```python
from build123d import *

# Parameters (mm, degrees)
SKETCH1_W           = 90
SKETCH1_H           = 30
SKETCH1_R           = 10.585
BOSS_EXTRUDE1_DEPTH = 80
SKETCH2_W           = 90
SKETCH2_H           = 30
BOSS_EXTRUDE2_DEPTH = 5
SKETCH3_W           = 90
SKETCH3_H           = 30
BOSS_EXTRUDE3_DEPTH = 5
SKETCH4_W           = 81.17
SKETCH4_H           = 74
CUT_EXTRUDE1_DEPTH  = 15


with BuildPart() as part:
    # Sketch1 → Boss-Extrude1 (new body)
    with BuildSketch(Plane(origin=(0, 0, 0), x_dir=(1, 0, 0), z_dir=(0, 1, 0))):
        with Locations((30, 0)):
            Rectangle(SKETCH1_W, SKETCH1_H)
        with Locations(Location((0, 0, 0), (0, 0, 270))):
            Circle(SKETCH1_R, mode=Mode.SUBTRACT)
        with Locations(Location((60, 0, 0), (0, 0, 270))):
            Circle(SKETCH1_R, mode=Mode.SUBTRACT)
        with Locations(Location((30, 0, 0), (0, 0, 270))):
            Circle(SKETCH1_R, mode=Mode.SUBTRACT)
    extrude(amount=BOSS_EXTRUDE1_DEPTH)

    # Sketch2 → Boss-Extrude2 (add)
    with BuildSketch(Plane(origin=(0, 80, 0), x_dir=(1, 0, 0), z_dir=(0, 1, 0))):
        with Locations((30, 0)):
            Rectangle(SKETCH2_W, SKETCH2_H)
    extrude(amount=BOSS_EXTRUDE2_DEPTH)

    # Sketch3 → Boss-Extrude3 (add)
    with BuildSketch(Plane.XZ):
        with Locations((30, 0)):
            Rectangle(SKETCH3_W, SKETCH3_H)
    extrude(amount=BOSS_EXTRUDE3_DEPTH)

    # Sketch4 → Cut-Extrude1 (cut)
    with BuildSketch(Plane(origin=(0, 0, -15), x_dir=(-1, 0, 0), z_dir=(0, 0, -1))):
        with Locations((-30, 40)):
            Rectangle(SKETCH4_W, SKETCH4_H)
    extrude(amount=-CUT_EXTRUDE1_DEPTH, mode=Mode.SUBTRACT)


solid = part.part
```
Geometry: final body of the model. Coordinates: model frame, mm. A direction names the side the tool comes from. Coordinates: 2 decimals unless noted, no trailing zeros. Write each loop counter-clockwise with the first axis right and the second up, starting at its lowest first coordinate (ties: lowest second). Pieces come first, ordered by that corner, then holes. Notation, with made-up numbers: M -20.75,59.5 L 9.25,59.5 A12 cw 9.25,70.5 Z; hole C 48,51 d3. An arc over 180 degrees is marked long. Answer as CSV lines item,"result". Start each with the question number.
Q1. Cut plane C-C on x = 25.5. Return the cut outline in (y, z).
Q2. Reachability of faces 5 (the flat face through (75, 41, 0)), 6 (the flat face through (0, 0, 0)), 7 (the flat face through (15, 41, 0)) from +Z, -Z, +X, -X, +Y, -Y: full face, straight path, thin tool, end or side. Return the list, or none.
Q3. Line query: line 1 (Y direction, x = -10.5, z = -0.5); line 2 (X direction, y = 4, z = -9.5) (3 decimals); line 3 (X direction, y = 37, z = 6.5). Output: solid intervals per line, ascending. Write a range as from..to.
Q4. Pin query (flat end, axial travel): P1, Ø9.5, axis at x = 44, y = 49.5, coming from the -Z side; P2, Ø3, axis at x = 55, y = 59, coming from the -Z side. Return the tip coordinate at first contact, or that it passes through.
Q5. Cut plane B-B on y = 43. Return the cut outline in (x, z) (3 decimals), then the cut area to 3 significant figures.
Q6. Cut plane A-A on z = 4.5. Return the cut outline in (x, y).
Q7. Mould query, pull axis Y, two halves, no side actions, for faces 1 (the flat face through (29, 41, 15)), 2 (the flat face through (29, -5, 0)), 3 (the flat face through (31, 3, -11)), 4 (the flat face through (30, 80, 0)). Classes: released by +Y, released by -Y, zero draft, split by the parting line, or undercut.
Findings below:
1,outline,"M -5,-15 L 3,-15 L 3,-9.58 L 0,-9.58 L 0,9.58 L 80,9.58 L 80,-9.58 L 77,-9.58 L 77,-15 L 85,-15 L 85,15 L -5,15 Z"
2,face 5,"+Z, -Z, +X, +Y, -Y"
2,face 6,"none"
2,face 7,"-Z"
3,line 1,"y = -5..0, 80..85"
3,line 2,"x = -15..-10.585, 70.585..75"
3,line 3,"x = -15..-8.35, 8.35..21.65, 38.35..51.65, 68.35..75"
4,P1,"stops at z = 0"
4,P2,"stops at z = 8.35"
5,outline,"M -15,-15 L -10.585,-15 L -10.585,0 A10.585 cw 10.585,0 L 19.415,0 A10.585 cw 40.585,0 L 49.415,0 A10.585 cw 70.585,0 L 70.585,-15 L 75,-15 L 75,15 L -15,15 Z"
5,area,"954 mm2"
6,outline,"M -15,-5 L 75,-5 L 75,85 L -15,85 Z; hole M -9.58,0 L 9.58,0 L 9.58,80 L -9.58,80 Z; hole M 20.42,0 L 39.58,0 L 39.58,80 L 20.42,80 Z; hole M 50.42,0 L 69.58,0 L 69.58,80 L 50.42,80 Z"
7,face 1,"zero draft"
7,face 2,"released by -Y"
7,face 3,"undercut"
7,face 4,"undercut"
